The model under review builds one solid part; all positions refer to its coordinate system, in mm. A direction names the side the tool comes from. Round coordinates to 2 decimals unless told otherwise and drop trailing zeros. Write each loop counter-clockwise with the first axis right and the second up, starting at its lowest first coordinate (ties: lowest second). Pieces come first, ordered by that corner, then holes. Notation, with made-up numbers: M -25,0.5 L 2,0.5 A26 cw 2,22.5 Z; hole C 22.5,-3 d2. An arc over 180 degrees is marked long. One line per item, written item: value. Start each with the question number.
1) Wall thickness on probe 1 along X at (y, z) = (35, 2.9); probe 2 along Y at (x, z) = (-41, 0.4); probe 3 along Y at (x, z) = (-93, 0.75): over which ranges is each line inside the solid? List them lowest first.
2) Tool access review of faces 4 (the face through (-25, 102, 1)), 5 (the face through (-75, 101, 1)), 6 (the face through (-89, 0, 1)), 7 (the face through (-102, 25, 1)): name each direction out of +Z, -Z, +X, -X, +Y, -Y from which nothing blocks a thin tool from reaching the whole face with its end or side.
3) Take a section at B-B, the plane z = 1.65. Write out the cut boundary in (x, y), and give its area (3 significant figures).
4) Take a section at A-A, the plane y = 35.5. Write out the cut boundary in (x, z).
5) Take a section at D-D, the plane x = -7. Write out the cut boundary in (y, z), and give its area (3 significant figures).
6) Take a section at C-C, the plane x = -45. Write out the cut boundary in (y, z).
7) For P1, Ø1.5, axis at y = 48, z = 2, coming from the -X side; P2, Ø1.5, axis at x = -16, z = 1.5, coming from the +Y side, all flat-tipped, find the tip position at first contact; note any pin that passes through.
8) Mouldability with a two-part tool opening along Y and no side actions: class faces 1 (the face through (-12, 0, 1)), 2 (the face through (-29, 51, 0)), 3 (the face through (-33.25, 50, 2)) as +Y half, -Y half, draft (parallel to the pull), parting line (faces both ways), or undercut.
Autodesk Inventor part; units mm, degrees
ref_plane "YZ Plane" through (0, 0, 0) normal (1, 0, 0) x (0, 1, 0)
ref_plane "XZ Plane" through (0, 0, 0) normal (0, 1, 0) x (-1, 0, 0)
ref_plane "XY Plane" through (0, 0, 0) normal (0, 0, 1) x (1, 0, 0)
sketch "Boceto1" plane through (0, 0, 0) normal (0, 0, 1) x (1, 0, 0)
  line L0 (0, 100) -> (0, 0)
  line L1 (-100, 25) -> (-100, 75)
  line L2 (-75, 0) -> (-75, -3)
  line L3 (-75, -3) -> (-25, -3)
  line L4 (-25, -3) -> (-25, 0)
  line L5 (0, 0) -> (-25, 0)
  line L6 (-103, 100) -> (-103, 75)
  line L7 (-103, 75) -> (-100, 75)
  line L8 (-103, 0) -> (-103, 25)
  line L9 (-103, 25) -> (-100, 25)
  line L10 (-103, 0) -> (-75, 0)
  line L11 (-75, 100) -> (-75, 103)
  line L12 (-75, 103) -> (-25, 103)
  line L13 (-25, 103) -> (-25, 100)
  line L14 (0, 100) -> (-25, 100)
  line L15 (-75, 100) -> (-103, 100)
  dimension "d1" = 100
  dimension "d4" = 50
  dimension "d5" = 25
  dimension "d7" = 25
  dimension "d8" = 25
  dimension "d9" = 3
  dimension "d10" = 3
  dimension "d11" = 100
  dimension "d13" = 50
  dimension "d14" = 3
extrude "Extrusión2" add sketch "Boceto1" along normal blind 3
sketch "Boceto2" plane through (0, 0, 3) normal (0, 0, 1) x (1, 0, 0)
  line L0 (-75, 100) -> (-103, 100)
  line L1 (-72.75, 69.75) -> (-33.25, 69.75)
  line L2 (-33.25, 69.75) -> (-33.25, 30.25)
  line L3 (-33.25, 30.25) -> (-72.75, 30.25)
  line L4 (-72.75, 30.25) -> (-72.75, 69.75)
  line L5 (-103, 25) -> (-103, 0)
  point P0 (0, 0)
  dimension "d37" = 39.5
  dimension "d38" = 39.5
  dimension "d39" = 30.25
  dimension "d40" = 30.25
extrude "Extrusión3" cut sketch "Boceto2" against normal blind 3
fillet "Empalme1" radius 2 4 edges at (-72.75, 69.75, 1.5) (-33.25, 69.75, 1.5) (-33.25, 30.25, 1.5) (-72.75, 30.25, 1.5)
properties part number "Control lateral"
Checked values:
1. probe 1: x = -100 to -72.75, -33.25 to 0
1. probe 2: y = -3 to 30.25, 69.75 to 103
1. probe 3: y = 0 to 100
2. face 4: +Z, -Z, +X, +Y
2. face 5: +Z, -Z, -X, +Y
2. face 6: +Z, -Z, -X, -Y
2. face 7: +Z, -Z, -X
3. outline: M -103,0 L -75,0 L -75,-3 L -25,-3 L -25,0 L 0,0 L 0,100 L -25,100 L -25,103 L -75,103 L -75,100 L -103,100 L -103,75 L -100,75 L -100,25 L -103,25 Z; hole M -72.75,32.25 A2 ccw -70.75,30.25 L -35.25,30.25 A2 ccw -33.25,32.25 L -33.25,67.75 A2 ccw -35.25,69.75 L -70.75,69.75 A2 ccw -72.75,67.75 Z
3. area: 8,890 mm2
4. outline: M -100,0 L -72.75,0 L -72.75,3 L -100,3 Z; M -33.25,0 L 0,0 L 0,3 L -33.25,3 Z
5. outline: M 0,0 L 100,0 L 100,3 L 0,3 Z
5. area: 300 mm2
6. outline: M -3,0 L 30.25,0 L 30.25,3 L -3,3 Z; M 69.75,0 L 103,0 L 103,3 L 69.75,3 Z
7. P1: stops at x = -100
7. P2: stops at y = 100
8. face 1: -Y half
8. face 2: draft
8. face 3: undercut
